```python
from build123d import *

# Parameters (mm, degrees)
F1_DEPTH = 6.35
F2_R     = 2.54


with BuildPart() as f1:
    # F0 (on Top) → F1 (new body)
    with BuildSketch(Plane.XY):
        with BuildLine():
            Line((-203.2, 0), (0, 0))
            Line((0, 0), (0, 19.05))
            Line((0, 19.05), (-203.2, 19.05))
            ThreePointArc((-203.2, 19.05), (-212.725, 9.525), (-203.2, 0))
        make_face()
    extrude(amount=F1_DEPTH)

    # F2
    f2_edges = [f1.edges().sort_by_distance(p)[0] for p in [
        (-101.6, 19.05, 0),
        (-101.6, 19.05, 6.35),
    ]]
    fillet(f2_edges, radius=F2_R)


solid = f1.part
```
The model under review builds one solid part; all positions refer to its coordinate system, in mm. Round coordinates to 2 decimals unless told otherwise and drop trailing zeros. Write each loop counter-clockwise with the first axis right and the second up, starting at its lowest first coordinate (ties: lowest second). Pieces come first, ordered by that corner, then holes. Notation, with made-up numbers: (54.5, 46) -> (64.5, 46) arc R18 ccw to (64.5, 50) -> close; hole circle Ø3 at (47, -15). An arc over 180 degrees is marked (long way). Use CSV: the item, a comma, the result in double quotes.
Q1. Consider section A-A (x = -176). Give the boundary of the cut face in (y, z), then the cut area to 3 significant figures.
Checks:
outline,"(0, 2.54) arc R2.54 ccw to (2.54, 0) -> (16.51, 0) arc R2.54 ccw to (19.05, 2.54) -> (19.05, 3.81) arc R2.54 ccw to (16.51, 6.35) -> (2.54, 6.35) arc R2.54 ccw to (0, 3.81) -> close"
area,"115 mm²"
Q2. Consider section B-B (z = 1.25). Give the boundary of the cut face in (x, y) (3 decimals).
Checks:
outline,"(-203.2, 0.352) -> (0, 0.352) -> (0, 18.698) -> (-203.2, 18.698) arc R9.173 ccw to start"
Q3. To check wall thickness, follow probe 1 along Y at (x, z) = (-168, 2); probe 2 along X at (y, z) = (4.5, 3.5); probe 3 along Z at (x, y) = (-105, 1.25). State the ranges of each line that lie inside material, in increasing order. Write a range as [from, to].
Checks:
probe 1,"[0.06, 18.99]"
probe 2,"[-211.29, 0]"
probe 3,"[0.35, 6]"
